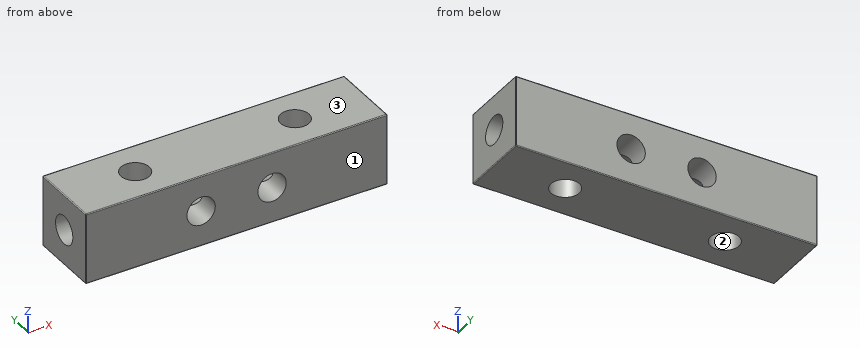
from build123d import *

# Parameters (mm, degrees)
SKETCH_1_W          = 8
SKETCH_1_H          = 8
EXTRUDE_1_DEPTH     = 34
FILLET_1_R          = 0.1
SKETCH_2_R          = 1.6
CUT_EXTRUDE_1_DEPTH = 35.467375879
SKETCH_3_R          = 1.6
CUT_EXTRUDE_2_DEPTH = 36.156791662
SKETCH_4_R          = 1.6
CUT_EXTRUDE_3_DEPTH = 36.156791662


with BuildPart() as part:
    # 草图1 → 凸台-拉伸1 (new body)
    with BuildSketch(Plane(origin=(0, 0, 0), x_dir=(0, 0, -1), z_dir=(1, 0, 0))):
        Rectangle(SKETCH_1_W, SKETCH_1_H)
    extrude(amount=EXTRUDE_1_DEPTH)

    # 圆角1
    fillet_1_edges = [part.edges().sort_by_distance(p)[0] for p in [
        (34, 0, 4),
        (34, -4, 0),
        (34, 0, -4),
        (0, -4, 0),
        (0, 0, 4),
        (0, 4, 0),
        (0, 0, -4),
        (17, -4, -4),
        (17, -4, 4),
        (17, 4, 4),
        (17, 4, -4),
        (34, 4, 0),
    ]]
    fillet(fillet_1_edges, radius=FILLET_1_R)

    # 草图2 → 切除-拉伸1 (cut, through all)
    with BuildSketch(Plane.ZY):
        Circle(SKETCH_2_R)
    extrude(amount=-CUT_EXTRUDE_1_DEPTH, mode=Mode.SUBTRACT)

    # 草图3 → 切除-拉伸2 (cut, through all)
    with BuildSketch(Plane.XY.offset(4)):
        with Locations((8, 0)):
            Circle(SKETCH_3_R)
        with Locations((26, 0)):
            Circle(SKETCH_3_R)
    extrude(amount=-CUT_EXTRUDE_2_DEPTH, mode=Mode.SUBTRACT)

    # 草图4 → 切除-拉伸3 (cut, through all)
    with BuildSketch(Plane(origin=(0, 4, 0), x_dir=(1, 0, 0), z_dir=(0, 1, 0))):
        with Locations(Location((21, 0, 0), (0, 0, 270))):
            Circle(SKETCH_4_R)
        with Locations(Location((13, 0, 0), (0, 0, 270))):
            Circle(SKETCH_4_R)
    extrude(amount=-CUT_EXTRUDE_3_DEPTH, mode=Mode.SUBTRACT)


solid = part.part
Work out the finished part from the listing and answer in its coordinate system (mm). Face numbers are marked on the shaded views. Coordinates: 2 decimals unless noted, no trailing zeros. Write each loop counter-clockwise with the first axis right and the second up, starting at its lowest first coordinate (ties: lowest second). Pieces come first, ordered by that corner, then holes. Notation, with made-up numbers: M 50.5,-29 L 104.5,-29 A19 ccw 104.5,6 Z; hole C 80,46.5 d2. An arc over 180 degrees is marked long. Write item = value, one per line.
1. The part is cut by section C-C (z = 3.5). Determine the outline of the cut face in (x, y), then the cut area to 3 significant figures.
Solution:
outline = M 0,-3.9 A0.1 ccw 0.1,-4 L 33.9,-4 A0.1 ccw 34,-3.9 L 34,3.9 A0.1 ccw 33.9,4 L 0.1,4 A0.1 ccw 0,3.9 Z; hole C 8,0 d3.2; hole C 26,0 d3.2
area = 256 mm2
2. The part is cut by section B-B (y = 3.5). Determine the outline of the cut face in (x, z), then the cut area to 3 significant figures.
Solution:
outline = M 0,-3.9 A0.1 ccw 0.1,-4 L 33.9,-4 A0.1 ccw 34,-3.9 L 34,3.9 A0.1 ccw 33.9,4 L 0.1,4 A0.1 ccw 0,3.9 Z; hole C 13,0 d3.2; hole C 21,0 d3.2
area = 256 mm2
3. The part is cut by section A-A (x = 5). Determine the outline of the cut face in (y, z).
Solution:
outline = M -4,-3.9 A0.1 ccw -3.9,-4 L 3.9,-4 A0.1 ccw 4,-3.9 L 4,3.9 A0.1 ccw 3.9,4 L -3.9,4 A0.1 ccw -4,3.9 Z; hole C 0,0 d3.2
4. Straight lines are drawn through the part: line 1 (X direction, y = 1.9, z = 0); line 2 (Z direction, x = 13, y = -1); line 3 (X direction, y = -3.25, z = 0.5). For each, find the intervals that lie inside material, in ascending order. Write a range as from..to.
Solution:
line_1 = 0..11.4, 14.6..19.4, 22.6..34
line_2 = -4..-1.6, 1.6..4
line_3 = 0..11.48, 14.52..19.48, 22.52..34
5. A flat-ended cylindrical pin translates along its axis: pin 1 (4 mm diameter, centred on x = 8, y = 0, fed in from -Z). Find the tip coordinate at first contact, or state that the pin passes through.
Solution:
pin_1 = -4
6. Determine the mould class of the marked faces 1, 2 and 3 for opening direction Y: released by +Y, released by -Y, zero draft, split by the parting line, or undercut.
Solution:
face_1 = released by -Y
face_2 = undercut
face_3 = zero draft
7. The part is cut by section D-D (z = 0.5). State how many separate pieces and enclosed holes the cut face has, then the cut area to 3 significant figures.
Solution:
separate_pieces = 6
enclosed_holes = 0
area = 138 mm2
